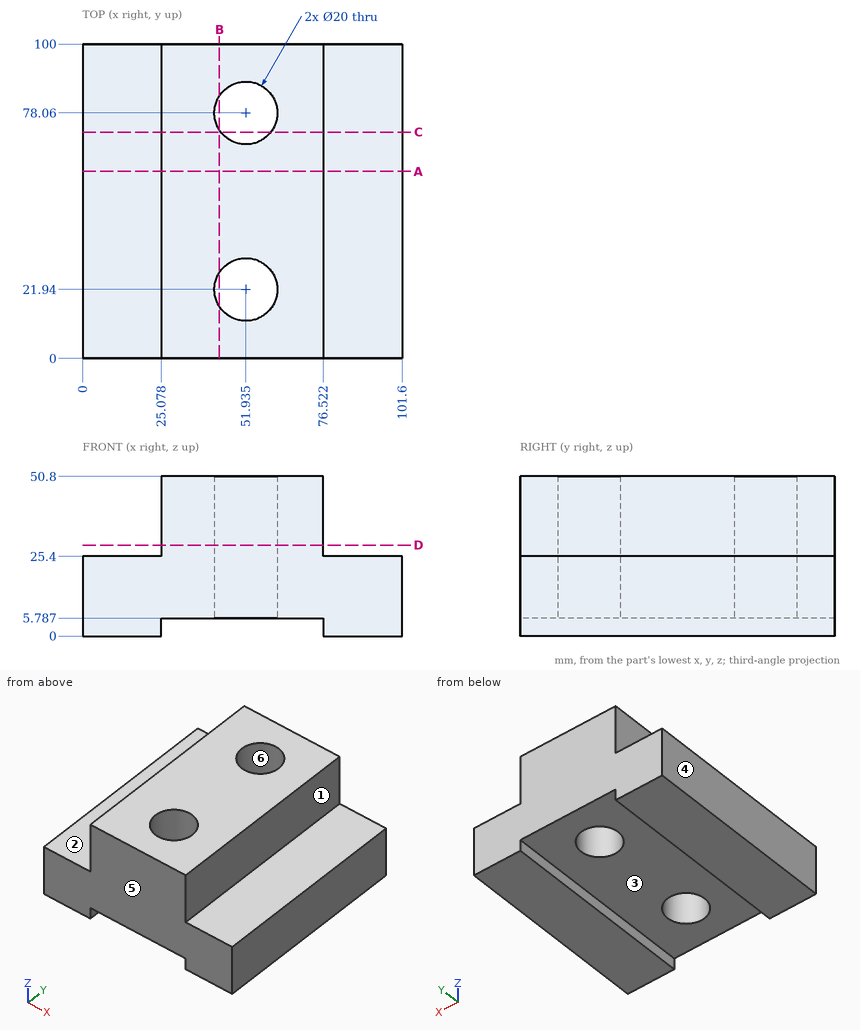
For this review, use the dimensioned drawing (mm, ordinates from the lowest corner) and the shaded views. A direction names the side the tool comes from. Coordinates: 2 decimals unless noted, no trailing zeros. Write each loop counter-clockwise with the first axis right and the second up, starting at its lowest first coordinate (ties: lowest second). Pieces come first, ordered by that corner, then holes. Notation, with made-up numbers: (25, -9) - (64, -9) arc R19 cw to (64, 8) - close; hole circle Ø2 at (-28, -8.75). An arc over 180 degrees is marked (long way). Answer in a Markdown table with one row per item. Add a question column.
Q1. Clearance check with flat-ended pins moving along their axes: pin 1 (1.5 mm diameter, centred on x = 57.5, y = 70, fed in from +Z); pin 2 (1.5 mm diameter, centred on x = 41.5, y = 52, fed in from -Z); pin 3 (12 mm diameter, centred on x = 51.93, y = 21.94, fed in from +Z); pin 4 (7.5 mm diameter, centred on x = 12, y = 31.5, fed in from +Z). State where each tip first meets the part, or that it passes through.
Q2. To check wall thickness, follow line 1 along Y through (x, z) = (58, 19); line 2 along Y through (x, z) = (55, 29); line 3 along X through (y, z) = (51, 44). State the ranges of each line that lie inside material, in increasing order. Write a range as from..to.
Q3. Consider section B-B on x = 43.5. Give the boundary of the cut face in (y, z).
Q4. Consider section D-D on z = 29. Give the boundary of the cut face in (x, y) (1 decimal).
Q5. For the marked faces 1, 2 and 3, list the 3-axis set-ups (+Z, -Z, +X, -X, +Y, -Y) from which the entire face can be reached by the end or side of a thin tool; tool diameter is ignored.
Q6. Consider section C-C on y = 72. Give the boundary of the cut face in (x, z), then the cut area to 3 significant figures.
Q7. Consider section A-A on y = 59.5. Give the boundary of the cut face in (x, z), then the cut area to 3 significant figures.
Q8. Draft analysis for pull direction X (two halves, no side actions). For the marked faces 4, 5 and 6, state which applies: +X half, -X half, draft (parallel to the pull), parting line (faces both ways), or undercut.
Answers below:
| question | item | result |
|---|---|---|
| 1 | pin 1 | z = 50.8 |
| 1 | pin 2 | z = 5.79 |
| 1 | pin 3 | through |
| 1 | pin 4 | z = 25.4 |
| 2 | line 1 | 0..13.99, 29.89..70.11, 86.01..100 |
| 2 | line 2 | 0..12.42, 31.46..68.54, 87.58..100 |
| 2 | line 3 | 25.08..76.52 |
| 3 | outline | (0, 5.79) - (16.57, 5.79) - (16.57, 50.8) - (0, 50.8) - close; (27.31, 5.79) - (72.69, 5.79) - (72.69, 50.8) - (27.31, 50.8) - close; (83.43, 5.79) - (100, 5.79) - (100, 50.8) - (83.43, 50.8) - close |
| 4 | outline | (25.1, 0) - (76.5, 0) - (76.5, 100) - (25.1, 100) - close; hole circle Ø20 at (51.9, 21.9); hole circle Ø20 at (51.9, 78.1) |
| 5 | face 1 | +Z, +X, +Y, -Y |
| 5 | face 2 | +Z, -X, +Y, -Y |
| 5 | face 3 | -Z, +Y, -Y |
| 6 | outline | (0, 0) - (25.08, 0) - (25.08, 5.79) - (43.98, 5.79) - (43.98, 50.8) - (25.08, 50.8) - (25.08, 25.4) - (0, 25.4) - close; (59.89, 5.79) - (76.52, 5.79) - (76.52, 0) - (101.6, 0) - (101.6, 25.4) - (76.52, 25.4) - (76.52, 50.8) - (59.89, 50.8) - close |
| 6 | area | 2,870 mm² |
| 7 | outline | (0, 0) - (25.08, 0) - (25.08, 5.79) - (76.52, 5.79) - (76.52, 0) - (101.6, 0) - (101.6, 25.4) - (76.52, 25.4) - (76.52, 50.8) - (25.08, 50.8) - (25.08, 25.4) - (0, 25.4) - close |
| 7 | area | 3,590 mm² |
| 8 | face 4 | -X half |
| 8 | face 5 | draft |
| 8 | face 6 | undercut |
